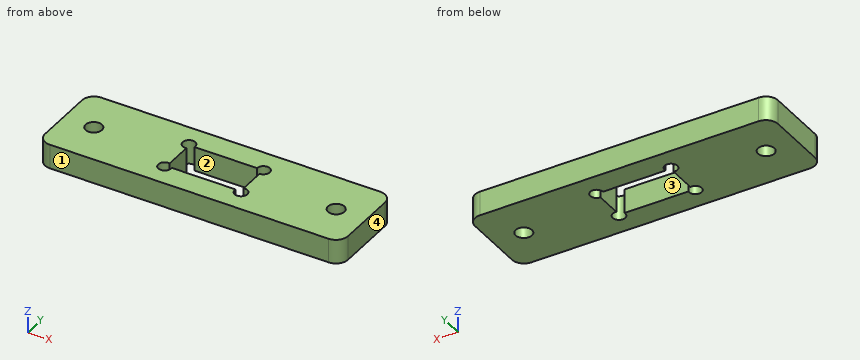
Autodesk Inventor part; units mm, degrees
ref_plane "YZ Plane" through (0, 0, 0) normal (1, 0, 0) x (0, 1, 0)
ref_plane "XZ Plane" through (0, 0, 0) normal (0, 1, 0) x (-1, 0, 0)
ref_plane "XY Plane" through (0, 0, 0) normal (0, 0, 1) x (1, 0, 0)
ref_plane "작업 평면1" through (80.2, 0, -34) normal (0, 0, -1) x (-1, 0, 0)
sketch "스케치1" plane through (80.2, 0, -34) normal (0, 0, -1) x (-1, 0, 0)
  line L0 (34.1, 0) -> (46.1, 0)
  line L1 (46.1, 0) -> (46.1, 6)
  line L2 (34.1, 6) -> (46.1, 6)
  line L3 (34.1, 0) -> (34.1, 6)
  line L4 (46.2, 6.1) -> (46.2, -0.1)
  line L5 (46.2, -0.1) -> (34, -0.1)
  line L6 (34, -0.1) -> (34, 6.1)
  line L7 (34, 6.1) -> (46.2, 6.1)
  line L8 (33.1, 0) -> (33.1, 6)
  line L9 (0, 6) -> (33.1, 6)
  line L10 (0, 0) -> (0, 6)
  line L11 (0, 0) -> (33.1, 0)
  circle A0 centre (20.1, 3) radius 1.35
  line L12 (47.1, 6) -> (47.1, 0)
  line L13 (47.1, 0) -> (80.2, 0)
  line L14 (80.2, 0) -> (80.2, 6)
  line L15 (47.1, 6) -> (80.2, 6)
  circle A1 centre (60.1, 3) radius 1.35
  line L16 (50.1, 10) -> (50.1, -4)
  line L17 (50.1, -4) -> (30.1, -4)
  line L18 (30.1, -4) -> (30.1, 10)
  line L19 (30.1, 10) -> (50.1, 10)
  line L20 (15.1, -4) -> (25.1, -4)
  line L21 (25.1, -4) -> (25.1, 10)
  line L22 (25.1, 10) -> (15.1, 10)
  line L23 (15.1, 10) -> (15.1, -4)
  line L24 (15.1, -4) -> (25.1, 10) construction
  line L25 (25.1, -4) -> (15.1, 10) construction
  line L26 (55.1, -4) -> (65.1, -4)
  line L27 (65.1, -4) -> (65.1, 10)
  line L28 (65.1, 10) -> (55.1, 10)
  line L29 (55.1, 10) -> (55.1, -4)
  line L30 (55.1, -4) -> (65.1, 10) construction
  line L31 (65.1, -4) -> (55.1, 10) construction
  line L32 (15.1, 10) -> (65.1, 10)
  line L33 (65.1, 10) -> (65.1, -4)
  line L34 (65.1, -4) -> (15.1, -4)
  line L35 (15.1, -4) -> (15.1, 10)
  circle A2 centre (34, 6.1) radius 1.05
  circle A3 centre (33.8, -0.3) radius 1.05
  circle A4 centre (46.4, -0.3) radius 1.05
  circle A5 centre (46.4, 6.3) radius 1.05
  point P0 (34, 0.7308)
  point P1 (34, 5.05)
  point P2 (35.05, 6.1)
  point P3 (45.3692, 6.1)
  point P4 (46.2, 5.2692)
  point P5 (46.2, 0.7308)
  point P6 (45.3692, -0.1)
  point P7 (34.8308, -0.1)
  point P8 (50.1, -4)
  dimension "d0" = 0.1
  dimension "d1" = 4
  dimension "d2" = 10
  dimension "d3" = 14
  dimension "d4" = 10
  dimension "d5" = 14
  dimension "d6" = 2.1
  dimension "d7" = 2.1
  dimension "d8" = 2.1
  dimension "d9" = 2.1
extrude "돌출1" add sketch "스케치1" along normal blind 4 contours L5 A4 L13 L16 L17 L18 L11 A3 | A3 L8 A2 L6 | A3 L11 L18 L9 A2 L8 | L4 A5 L12 A4 | A2 L9 L18 L19 L16 L15 A5 L7 | L12 A5 L15 L16 L13 A4 | L18 L34 L21 L11 | L11 L21 L9 L18 | L16 L15 L29 L13 | L13 L29 L34 L16 | L21 L20 L23 L11 | L11 L23 L9 L21 | L9 L21 L32 L18 | L29 L15 L27 L13 | L13 L27 L26 L29 | L16 L32 L29 L15 | L9 L23 L22 L21 | L29 L28 L27 L15
fillet "모깎기1" radius 2 4 edges at (15.1, -4, -36) (15.1, 10, -36) (65.1, -4, -36) (65.1, 10, -36)
properties part number "zig8"
Can you work these out from the model? Positions are in its coordinate system, mm. Face numbers are marked on the shaded views. Give positions to 0.01 mm unless a question says otherwise; leave off trailing zeros. Loops run counter-clockwise (first coordinate to the right, second up) from the corner with the lowest first, then second, coordinate; pieces in that order, holes last. Notation, with made-up numbers: M 10,83.5 L 29,83.5 A23 ccw 29,110.5 Z; hole C 75.25,-1 d8. An arc over 180 degrees is marked long. Use CSV: the item, a comma, the result in double quotes. Start each with the question number.
1. For P1, Ø2, axis at x = 60.1, y = 3, coming from the +Z side, with a flat end and sliding along its axis, tell me the tip position at first contact or that it passes through.
2. Imagine slicing it at D-D, the plane x = 60.1. Write out the boundary of the cut face in (y, z).
3. Imagine slicing it at B-B, the plane y = 3. Write out the boundary of the cut face in (x, z), plus the area to 3 significant figures.
4. If I drill on L1, parallel to X at y = -0.3, z = -36.3; L2, parallel to Y at x = 33.8, z = -37.1; L3, parallel to Y at x = 20.1, z = -36.6, over which ranges is the centre line in solid material (lowest first)?
5. Imagine slicing it at C-C, the plane z = -34.45. Write out the boundary of the cut face in (x, y).
6. Imagine slicing it at A-A, the plane x = 36. Write out the boundary of the cut face in (y, z).
7. If we mould it in two halves opening along X, with no side actions, what happens to the marked faces 1, 2, 3 and 4? For each: released by +X, released by -X, zero draft, split by the parting line, or undercut.
Response values:
1,P1,"through"
2,outline,"M -4,-38 L 1.65,-38 L 1.65,-34 L -4,-34 Z; M 4.35,-38 L 10,-38 L 10,-34 L 4.35,-34 Z"
3,outline,"M 15.1,-38 L 18.75,-38 L 18.75,-34 L 15.1,-34 Z; M 21.45,-38 L 34,-38 L 34,-34 L 21.45,-34 Z; M 46.2,-38 L 58.75,-38 L 58.75,-34 L 46.2,-34 Z; M 61.45,-38 L 65.1,-38 L 65.1,-34 L 61.45,-34 Z"
3,area,"130 mm^2"
4,L1,"15.1 to 32.75, 34.85 to 45.35, 47.45 to 65.1"
4,L2,"-4 to -1.35, 0.75 to 5.25, 7.35 to 10"
4,L3,"-4 to 1.65, 4.35 to 10"
5,outline,"M 15.1,-2 A2 ccw 17.1,-4 L 63.1,-4 A2 ccw 65.1,-2 L 65.1,8 A2 ccw 63.1,10 L 17.1,10 A2 ccw 15.1,8 Z; hole C 20.1,3 d2.7; hole M 34,0.73 A1.05 ccw long 34.83,-0.1 L 45.37,-0.1 A1.05 ccw long 46.2,0.73 L 46.2,5.05 A1.05 ccw long 45.15,6.1 L 34.83,6.1 A1.05 ccw long 34,5.27 Z; hole C 60.1,3 d2.7"
6,outline,"M -4,-38 L -0.1,-38 L -0.1,-34 L -4,-34 Z; M 6.1,-38 L 10,-38 L 10,-34 L 6.1,-34 Z"
7,face 1,"zero draft"
7,face 2,"undercut"
7,face 3,"undercut"
7,face 4,"released by +X"
